Read the model definition and answer for the solid it produces. Units are mm, in the model's axes. Coordinates: 2 decimals unless noted, no trailing zeros. Write each loop counter-clockwise with the first axis right and the second up, starting at its lowest first coordinate (ties: lowest second). Pieces come first, ordered by that corner, then holes.
(1) The mould has two halves that part along X. Classify faces 1 (the flat face through (0, 113, 12)), 2 (the flat face through (0, 122.668, 0)), 3 (the flat face through (0, 113, -12)), 4 (the conical face through (-19.42, 47.06, 6.11)): +X half, -X half, draft (parallel to the pull), parting line (faces both ways), or undercut.
(2) Given pin 1 (6 mm diameter, centred on x = 3.5, z = -7.5, fed in from -Y); pin 2 (3 mm diameter, centred on x = 18, y = 7, fed in from -Z); pin 3 (6 mm diameter, centred on x = 13, y = -10.5, fed in from -Z); pin 4 (5 mm diameter, centred on x = 2, y = -11, fed in from +Z), each flat-ended and moving along its own axis, determine where each tip first touches the part or whether it passes through.
(3) Section A-A on y = 68 is taken. Write down the section's boundary in (x, z), then the cut area to 3 significant figures.
(4) Find the intervals of material crossed by probe 1 along Z at (x, y) = (-3.5, -22); probe 2 along Y at (x, z) = (-2, 11); probe 3 along X at (y, z) = (67.5, 7), in increasing order.
from build123d import *

# Parameters (mm, degrees)
ENL_V_MAT_EXTRU_1_DEPTH      = 7.5
ENL_V_MAT_EXTRU_1_DEPTH_BACK = 7.5
BOSS_EXTRU_1_REACH           = 27.5
ECHELLE1_SCALE               = 1.6


with BuildPart() as part:
    # Esquisse1 → R_volution1 (revolve)
    with BuildSketch(Plane.XY):
        with BuildLine():
            Line((0, 0), (0, 100))
            Line((0, 100), (-18, 100))
            Line((-18, 100), (-7.593007693, 6.792401612))
            ThreePointArc((-7.593007693, 6.792401612), (-5.093880777, 1.945904787), (0, 0))
        make_face()
    revolve(axis=Axis((0, 0, 0), (0, 1, 0)))

    # Esquisse2 → Enl_v. mat.-Extru.1 (cut, two sides)
    with BuildSketch(Plane.XY) as enl_v_mat_extru_1_sk:
        with BuildLine():
            Line((-13.5, 100), (13.5, 100))
            add(Edge.make_bspline(
                [(-13.5, 100), (-13.291113541, 83.520875666), (13.291113541, 83.520875666), (13.5, 100)],
                knots=[0, 0, 0, 0, 1, 1, 1, 1], degree=3))
        make_face()
    extrude(amount=ENL_V_MAT_EXTRU_1_DEPTH, mode=Mode.SUBTRACT)
    extrude(enl_v_mat_extru_1_sk.sketch, amount=-ENL_V_MAT_EXTRU_1_DEPTH_BACK, mode=Mode.SUBTRACT)

    # Esquisse3 → Boss.-Extru.1 (add, up to next)
    with BuildSketch(Plane.XY.offset(-7.5), mode=Mode.PRIVATE) as boss_extru_1_sk1:
        with BuildLine():
            Line((-5, 100), (5, 100))
            add(Edge.make_bspline(
                [(-5, 100), (0, 91.498247822), (5, 100)],
                knots=[0, 0, 0, 1, 1, 1], degree=2))
        make_face()
    boss_extru_1_tool1 = extrude(boss_extru_1_sk1.sketch, amount=BOSS_EXTRU_1_REACH, mode=Mode.PRIVATE) - part.part
    add(boss_extru_1_tool1.solids().sort_by_distance((0, 98.29965, -7.5))[0])


with BuildPart() as part_1:
    # Echelle1: scaled about (-4e-09, 62.219241992, 3e-09)
    add(part.part.scale(ECHELLE1_SCALE).moved(Location((2e-09, -37.331545195, -2e-09))))


solid = part_1.part
Response:
1. face 1: undercut
1. face 2: draft
1. face 3: undercut
1. face 4: parting line
2. pin 1: stops at y = -36.13
2. pin 2: passes through
2. pin 3: stops at z = -9.74
2. pin 4: stops at z = 14.1
3. outline: circle Ø45.39 at (0, 0)
3. area: 1,620 mm2
4. probe 1: z = -12.15 to 12.15
4. probe 2: y = -30.05 to 102.97, 116.29 to 122.67
4. probe 3: x = -21.53 to 21.53
